from build123d import *

# Parameters (mm, degrees)
SKETCH1_W           = 26
SKETCH1_H           = 25
BOSS_EXTRUDE1_DEPTH = 1
SKETCH2_R           = 12.5
BOSS_EXTRUDE2_DEPTH = 54
SKETCH3_R           = 6
CUT_EXTRUDE1_DEPTH  = 56


with BuildPart() as part:
    # Sketch1 → Boss-Extrude1 (new body)
    with BuildSketch(Plane.XY):
        Rectangle(SKETCH1_W, SKETCH1_H)
    extrude(amount=BOSS_EXTRUDE1_DEPTH)

    # Sketch2 → Boss-Extrude2 (add)
    with BuildSketch(Plane.XY.offset(1)):
        Circle(SKETCH2_R)
    extrude(amount=BOSS_EXTRUDE2_DEPTH)

    # Sketch3 → Cut-Extrude1 (cut, through all)
    with BuildSketch(Plane(origin=(0, 0, 0), x_dir=(-1, 0, 0), z_dir=(0, 0, -1))):
        Circle(SKETCH3_R)
    extrude(amount=-CUT_EXTRUDE1_DEPTH, mode=Mode.SUBTRACT)


solid = part.part
The listing builds one solid part. Answer for the finished solid, in the listing's coordinates (mm). A direction names the side the tool comes from. Give positions to 0.01 mm unless a question says otherwise; leave off trailing zeros. Order: outer loops, then holes, each group sorted by start corner. A loop starts at its lowest first (then second) coordinate and runs counter-clockwise, first axis right, second up. Notation, with made-up numbers: (-15.5, 78.5) -> (8.5, 78.5) arc R22 ccw to (8.5, 100.5) -> close; hole circle Ø5 at (70.25, -16). An arc over 180 degrees is marked (long way). Put each result on its own line as item: value.
Item 1: Straight lines are drawn through the part: line 1 (Y direction, x = 0, z = 25.5); line 2 (Y direction, x = 5, z = 25.5); line 3 (Z direction, x = 10.75, y = -11). For each, find the intervals that lie inside material, in ascending order.
Established:
line 1: y = -12.5 to -6, 6 to 12.5
line 2: y = -11.46 to -3.32, 3.32 to 11.46
line 3: z = 0 to 1
Item 2: A cutting plane is placed at A-A on y = 0. Give the vertices of the cut face in (x, z), plus the area to 3 significant figures.
Established:
outline: (-13, 0) -> (-6, 0) -> (-6, 55) -> (-12.5, 55) -> (-12.5, 1) -> (-13, 1) -> close; (6, 0) -> (13, 0) -> (13, 1) -> (12.5, 1) -> (12.5, 55) -> (6, 55) -> close
area: 716 mm^2
Item 3: For faces 1 (the face through (11.923, 3.755, 27.622)), 2 (the face through (-12.8, -0.9, 1)), 3 (the face through (-0.2, 12.5, 0.5)), determine the directions among +Z, -Z, +X, -X, +Y, -Y from which every point of the face is accessible in a straight line to the end or side of a thin tool.
Established:
face 1: +Z
face 2: +Z, -X
face 3: +Z, -Z, +X, -X, +Y
Item 4: Given P1, Ø3, axis at x = 4, z = 8.5, coming from the +Y side; P2, Ø10, axis at y = 4, z = 45.5, coming from the +X side; P3, Ø5, axis at y = -5.5, z = 13, coming from the -X side, each flat-ended and moving along its own axis, determine where each tip first touches the part or whether it passes through.
Established:
P1: stops at y = 12.25
P2: stops at x = 12.5
P3: stops at x = -12.13
Item 5: A cutting plane is placed at B-B on x = -3.5. Give the vertices of the cut face in (y, z), plus the area to 3 significant figures.
Established:
outline: (-12.5, 0) -> (-4.87, 0) -> (-4.87, 55) -> (-12, 55) -> (-12, 1) -> (-12.5, 1) -> close; (4.87, 0) -> (12.5, 0) -> (12.5, 1) -> (12, 1) -> (12, 55) -> (4.87, 55) -> close
area: 785 mm^2
Item 6: A cutting plane is placed at C-C on z = 48. Give the vertices of the cut face in (x, y), plus the area to 3 significant figures.
Established:
outline: circle Ø25 at (0, 0); hole circle Ø12 at (0, 0)
area: 378 mm^2
Item 7: For a pull along X with two mould halves and no side action, classify faces 4 (the face through (-13, -0.2, 0.5)), 5 (the face through (6, 0, 27)), 6 (the face through (12.7, 1, 1)) as released by +X, released by -X, zero draft, split by the parting line, or undercut.
Established:
face 4: released by -X
face 5: undercut
face 6: zero draft
